Verification items for the finished model (mm, model axes). Face numbers are marked on the shaded views. A direction names the side the tool comes from. Give positions to 0.01 mm unless a question says otherwise; leave off trailing zeros. Write each loop counter-clockwise with the first axis right and the second up, starting at its lowest first coordinate (ties: lowest second). Pieces come first, ordered by that corner, then holes.
from build123d import *

# Parameters (mm, degrees)
F2_R     = 7.5
F3_DEPTH = 65.001
F4_R     = 7.5
F5_DEPTH = 8
F6_SIZE2 = 2.8867513459
F6_SIZE  = 5


with BuildPart() as f1:
    # F0 (on Front) → F1 (revolve)
    with BuildSketch(Plane.XZ):
        Polygon((-29, 13.2), (-29, 0), (36, 0), (36, 13.2), (0, 13.2), (0, 15.6), (-10, 15.6), (-10, 13.2), align=None)
    revolve(axis=Axis((5.8021252709, 0, 0), (1, 0, 0)))

    # F2 (on face) → F3 (cut, through all)
    with BuildSketch(Plane.YZ.offset(36)):
        Circle(F2_R)
    extrude(amount=-F3_DEPTH, mode=Mode.SUBTRACT)

    # F4 (on Right) → F5 (join)
    with BuildSketch(Plane.YZ):
        with BuildLine():
            Line((-17, 4.1533119315), (-17, -4.1533119315))
            ThreePointArc((-17, -4.1533119315), (-15.1554445662, -8.75), (-12.0968736425, -12.6457758986))
            Line((-12.0968736425, -12.6457758986), (-4.9031263575, -16.7990878301))
            ThreePointArc((-4.9031263575, -16.7990878301), (0, -17.5), (4.9031263575, -16.7990878301))
            Line((4.9031263575, -16.7990878301), (12.0968736425, -12.6457758986))
            ThreePointArc((12.0968736425, -12.6457758986), (15.1554445662, -8.75), (17, -4.1533119315))
            Line((17, -4.1533119315), (17, 4.1533119315))
            ThreePointArc((17, 4.1533119315), (15.1554445662, 8.75), (12.0968736425, 12.6457758986))
            Line((12.0968736425, 12.6457758986), (4.9031263575, 16.7990878301))
            ThreePointArc((4.9031263575, 16.7990878301), (0, 17.5), (-4.9031263575, 16.7990878301))
            Line((-4.9031263575, 16.7990878301), (-12.0968736425, 12.6457758986))
            ThreePointArc((-12.0968736425, 12.6457758986), (-15.1554445662, 8.75), (-17, 4.1533119315))
        make_face()
        Circle(F4_R, mode=Mode.SUBTRACT)
        with BuildLine():
            Line((-17, 9.8149545762), (-17, 4.1533119315))
            ThreePointArc((-17, 4.1533119315), (-15.1554445662, 8.75), (-12.0968736425, 12.6457758986))
            Line((-12.0968736425, 12.6457758986), (-17, 9.8149545762))
        make_face()
        with BuildLine():
            Line((-17, -4.1533119315), (-17, -9.8149545762))
            Line((-17, -9.8149545762), (-12.0968736425, -12.6457758986))
            ThreePointArc((-12.0968736425, -12.6457758986), (-15.1554445662, -8.75), (-17, -4.1533119315))
        make_face()
        with BuildLine():
            ThreePointArc((4.9031263575, -16.7990878301), (0, -17.5), (-4.9031263575, -16.7990878301))
            Line((-4.9031263575, -16.7990878301), (0, -19.6299091524))
            Line((0, -19.6299091524), (4.9031263575, -16.7990878301))
        make_face()
        with BuildLine():
            ThreePointArc((17, -4.1533119315), (15.1554445662, -8.75), (12.0968736425, -12.6457758986))
            Line((12.0968736425, -12.6457758986), (17, -9.8149545762))
            Line((17, -9.8149545762), (17, -4.1533119315))
        make_face()
        with BuildLine():
            Line((17, 9.8149545762), (12.0968736425, 12.6457758986))
            ThreePointArc((12.0968736425, 12.6457758986), (15.1554445662, 8.75), (17, 4.1533119315))
            Line((17, 4.1533119315), (17, 9.8149545762))
        make_face()
        with BuildLine():
            Line((0, 19.6299091524), (-4.9031263575, 16.7990878301))
            ThreePointArc((-4.9031263575, 16.7990878301), (0, 17.5), (4.9031263575, 16.7990878301))
            Line((4.9031263575, 16.7990878301), (0, 19.6299091524))
        make_face()
    extrude(amount=-F5_DEPTH)

    # F6
    f6_edges = [f1.edges().sort_by_distance(p)[0] for p in [
        (-29, -7.5, 0),
    ]]
    chamfer(f6_edges, length=F6_SIZE, length2=F6_SIZE2)


solid = f1.part
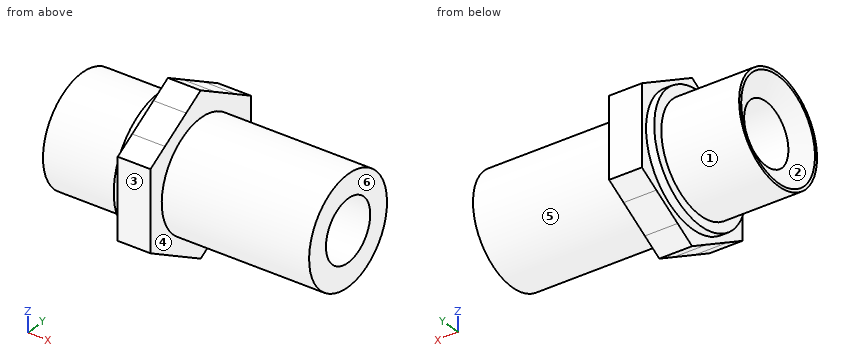
Item 1: Sectioned sample at A-A on z = 0. Record the cut outline in (x, y), then the cut area to 3 significant figures.
Answer key:
outline: (-29, -13.2) - (-10, -13.2) - (-10, -15.6) - (-8, -15.6) - (-8, -17) - (0, -17) - (0, -13.2) - (36, -13.2) - (36, -7.5) - (-26.11, -7.5) - (-29, -12.5) - close; (-29, 12.5) - (-26.11, 7.5) - (36, 7.5) - (36, 13.2) - (0, 13.2) - (0, 17) - (-8, 17) - (-8, 15.6) - (-10, 15.6) - (-10, 13.2) - (-29, 13.2) - close
area: 797 mm2
Item 2: Release check for a two-part mould opening along Y. For the marked faces 1, 2, 3 and 4 record: released by +Y, released by -Y, zero draft, split by the parting line, or undercut.
Answer key:
face 1: split by the parting line
face 2: undercut
face 3: released by -Y
face 4: zero draft
Item 3: Sectioned sample at C-C on x = 17. Record the cut outline in (y, z), then the cut area to 3 significant figures.
Answer key:
outline: circle Ø26.4 at (0, 0); hole circle Ø15 at (0, 0)
area: 371 mm2
Item 4: Depth check by flat-ended pin: pin 1 (2 mm diameter, centred on x = 0, y = -12.5, fed in from -Z); pin 2 (8 mm diameter, centred on x = 12, y = -1, fed in from -Z); pin 3 (12 mm diameter, centred on x = -17.5, z = 6.5, fed in from +Y). Enter the tip coordinate at first touch or a pass-through.
Answer key:
pin 1: stops at z = -12.99
pin 2: stops at z = -13.2
pin 3: stops at y = 13.19
Item 5: Set-up check for the marked faces 5 and 6: record each of +Z, -Z, +X, -X, +Y, -Y from which the full face is reachable in a straight line by a thin tool's end or side.
Answer key:
face 5: +X
face 6: +Z, -Z, +X, +Y, -Y
Item 6: Sectioned sample at B-B on x = -7. Record the cut outline in (y, z).
Answer key:
outline: (-17, -9.81) - (0, -19.63) - (17, -9.81) - (17, 9.81) - (0, 19.63) - (-17, 9.81) - close; hole circle Ø15 at (0, 0)
Item 7: Scan lines: line 1 along Z through (x, y) = (11.5, 0); line 2 along Z through (x, y) = (-3, 0); line 3 along X through (y, z) = (10.5, -11.5). Record each from-to range of solid material in increasing order.
Answer key:
line 1: z = -13.2 to -7.5, 7.5 to 13.2
line 2: z = -19.63 to -7.5, 7.5 to 19.63
line 3: x = -10 to 0
